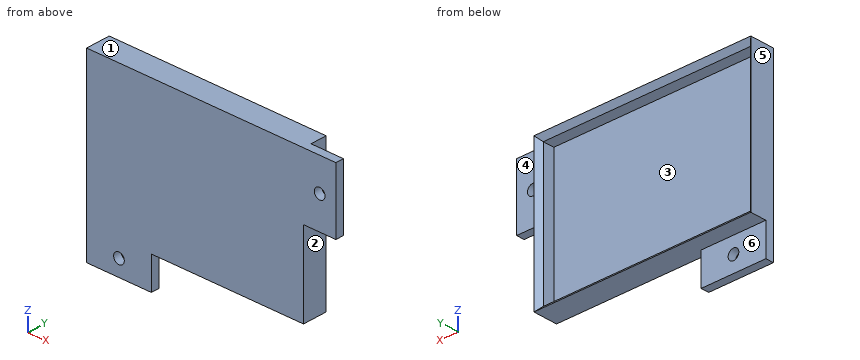
```python
from build123d import *

# Parameters (mm, degrees)
SKETCH1_W            = 134
SKETCH1_H            = 91.68
BOSS_EXTRUDE1_DEPTH  = 5
SKETCH2_W            = 40
SKETCH2_H            = 20
SKETCH2_W_2          = 20
SKETCH2_H_2          = 40
BOSS_EXTRUDE2_DEPTH  = 5
M6_CLEARANCE_HOLE1_D = 6.6
SKETCH6_W            = 134
SKETCH6_H            = 91.68
SKETCH6_W_2          = 128
SKETCH6_H_2          = 85.68
BOSS_EXTRUDE3_DEPTH  = 10
CHAMFER1_SIZE        = 3


with BuildPart() as part:
    # Sketch1 → Boss-Extrude1 (new body)
    with BuildSketch(Plane(origin=(0, 0, 0), x_dir=(1, 0, 0), z_dir=(0, 1, 0))):
        Rectangle(SKETCH1_W, SKETCH1_H)
    extrude(amount=BOSS_EXTRUDE1_DEPTH)

    # Sketch2 → Boss-Extrude2 (add)
    with BuildSketch(Plane(origin=(0, 0, 0), x_dir=(1, 0, 0), z_dir=(0, 1, 0))):
        with Locations((-47, 55.84)):
            Rectangle(SKETCH2_W, SKETCH2_H)
        with Locations((77, -25.84)):
            Rectangle(SKETCH2_W_2, SKETCH2_H_2)
    extrude(amount=BOSS_EXTRUDE2_DEPTH)

    # M6 Clearance Hole1 (through all)
    with Locations(Plane(origin=(0, 5, 0), x_dir=(1, 0, 0), z_dir=(0, 1, 0))):
        with Locations((-47, 55.84), (77, -25.84)):
            Hole(M6_CLEARANCE_HOLE1_D / 2)

    # Sketch6 → Boss-Extrude3 (add)
    with BuildSketch(Plane(origin=(0, 5, 0), x_dir=(1, 0, 0), z_dir=(0, 1, 0))):
        Rectangle(SKETCH6_W, SKETCH6_H)
        Rectangle(SKETCH6_W_2, SKETCH6_H_2, mode=Mode.SUBTRACT)
    extrude(amount=BOSS_EXTRUDE3_DEPTH)

    # Chamfer1
    chamfer1_edges = [part.edges().sort_by_distance(p)[0] for p in [
        (-64, 15, 0),
        (0, 15, 42.84),
        (64, 15, 0),
        (0, 15, -42.84),
    ]]
    chamfer(chamfer1_edges, length=CHAMFER1_SIZE - 0.0001)  # a hair under: the kernel refuses the full size


solid = part.part
```
Input: part model. Units: mm. Frame: model coordinates. Face numbers are marked on the shaded views. A direction names the side the tool comes from. Give positions to 0.01 mm unless a question says otherwise; leave off trailing zeros. Order: outer loops, then holes, each group sorted by start corner. A loop starts at its lowest first (then second) coordinate and runs counter-clockwise, first axis right, second up.
1. Pin query (flat end, axial travel): pin 1 (6 mm diameter, centred on y = 6.5, z = 7, fed in from +X); pin 2 (6 mm diameter, centred on y = 8, z = -22.5, fed in from +X); pin 3 (10.5 mm diameter, centred on x = -47, z = -55.84, fed in from +Y); pin 4 (3.5 mm diameter, centred on x = -9, y = 7, fed in from -Z). Return the tip coordinate at first contact, or that it passes through.
Derived:
pin 1: stops at x = 87
pin 2: stops at x = 67
pin 3: stops at y = 5
pin 4: stops at z = -45.84
2. Mould query, pull axis Z, two halves, no side actions, for the marked faces 1, 2 and 3. Classes: released by +Z, released by -Z, zero draft, split by the parting line, or undercut.
Derived:
face 1: released by +Z
face 2: zero draft
face 3: undercut
3. Reachability of the marked faces 4, 5 and 6 from +Z, -Z, +X, -X, +Y, -Y: full face, straight path, thin tool, end or side. Return the list, or none.
Derived:
face 4: +Z, -Z, +X, +Y
face 5: +Z, -Z, -X, +Y, -Y
face 6: -Z, +X, -X, +Y
4. Section D-D on y = 2. Return the cut outline in (x, z).
Derived:
outline: (-67, -65.84) - (-27, -65.84) - (-27, -45.84) - (67, -45.84) - (67, 5.84) - (87, 5.84) - (87, 45.84) - (-67, 45.84) - close; hole circle Ø6.6 at (-47, -55.84); hole circle Ø6.6 at (77, 25.84)
5. Section C-C on y = 10. Return the cut outline in (x, z).
Derived:
outline: (-67, -45.84) - (67, -45.84) - (67, 45.84) - (-67, 45.84) - close; hole (-64, -42.84) - (64, -42.84) - (64, 42.84) - (-64, 42.84) - close
6. Section A-A on x = 77. Return the cut outline in (y, z), and give its area (3 significant figures).
Derived:
outline: (0, 5.84) - (5, 5.84) - (5, 22.54) - (0, 22.54) - close; (0, 29.14) - (5, 29.14) - (5, 45.84) - (0, 45.84) - close
area: 167 mm2
7. Material intervals for L1, parallel to Z at x = 44, y = 9.25; L2, parallel to X at y = 1.4, z = 25.84; L3, parallel to X at y = 11.5, z = 4, sorted ascending.
Derived:
L1: z = -45.84 to -42.84, 42.84 to 45.84
L2: x = -67 to 73.7, 80.3 to 87
L3: x = -67 to -64, 64 to 67
